from build123d import *

# Parameters (mm, degrees)
SKETCH_1_R          = 28.4
EXTRUDE_1_DEPTH     = 6
SKETCH_2_R          = 15
EXTRUDE_2_DEPTH     = 20.4
SKETCH_3_R          = 7
CUT_EXTRUDE_1_DEPTH = 54.68780863
SKETCH_4_W          = 5
SKETCH_4_H          = 2.1
CUT_EXTRUDE_2_DEPTH = 54.68780863
SKETCH_5_R          = 2.6
CUT_EXTRUDE_3_DEPTH = 52.005693755


with BuildPart() as part:
    # 草图1 → 凸台-拉伸1 (new body)
    with BuildSketch(Plane.XY):
        with Locations((0, 8.733014899)):
            Circle(SKETCH_1_R)
    extrude(amount=EXTRUDE_1_DEPTH)

    # 草图2 → 凸台-拉伸2 (add)
    with BuildSketch(Plane.XY.offset(6)):
        with Locations((0, 8.733014899)):
            Circle(SKETCH_2_R)
    extrude(amount=EXTRUDE_2_DEPTH)

    # 草图3 → 切除-拉伸1 (cut, through all)
    with BuildSketch(Plane.XY.offset(26.4)):
        with Locations((0, 8.733014899)):
            Circle(SKETCH_3_R)
    extrude(amount=-CUT_EXTRUDE_1_DEPTH, mode=Mode.SUBTRACT)

    # 草图4 → 切除-拉伸2 (cut, through all)
    with BuildSketch(Plane.XY.offset(26.4)):
        with Locations((0, 16.321363314)):
            Rectangle(SKETCH_4_W, SKETCH_4_H)
    extrude(amount=-CUT_EXTRUDE_2_DEPTH, mode=Mode.SUBTRACT)

    # 草图5 → 切除-拉伸3 (cut, through all)
    with BuildSketch(Plane.XY.offset(6)):
        with Locations((0, 32.483014899)):
            Circle(SKETCH_5_R)
        with Locations((20.56810334, 20.608014899)):
            Circle(SKETCH_5_R)
        with Locations((20.56810334, -3.141985101)):
            Circle(SKETCH_5_R)
        with Locations((0, -15.016985101)):
            Circle(SKETCH_5_R)
        with Locations((-20.56810334, -3.141985101)):
            Circle(SKETCH_5_R)
        with Locations((-20.56810334, 20.608014899)):
            Circle(SKETCH_5_R)
    extrude(amount=-CUT_EXTRUDE_3_DEPTH, mode=Mode.SUBTRACT)


solid = part.part
Design review of the part built by this model. Coordinates are the model's own, in mm. A direction names the side the tool comes from. Give positions to 0.01 mm unless a question says otherwise; leave off trailing zeros. Loops run counter-clockwise (first coordinate to the right, second up) from the corner with the lowest first, then second, coordinate; pieces in that order, holes last. Notation, with made-up numbers: M 17.25,-21 L 31.25,-21 A36 ccw 31.25,13 Z; hole C 64,66 d3. An arc over 180 degrees is marked long. Answer as a JSON object with one key per item and string values.
Item 1: Wall thickness on line 1 along Y through (x, z) = (0, 3.4); line 2 along Y through (x, z) = (0, 7.5); line 3 along X through (y, z) = (21, 2): over which ranges is each line inside the solid? List them lowest first.
Output values:
{"line 1": "y = -19.67 to -17.62, -12.42 to 1.73, 17.37 to 29.88, 35.08 to 37.13", "line 2": "y = -6.27 to 1.73, 17.37 to 23.73", "line 3": "x = -25.61 to -23.14, -18 to 18, 23.14 to 25.61"}
Item 2: We need section C-C (x = 6). State the section outline as (y, z) points, and give its area (3 significant figures).
Output values:
{"outline": "M -19.03,0 L 5.13,0 L 5.13,26.4 L -5.01,26.4 L -5.01,6 L -19.03,6 Z; M 12.34,0 L 36.49,0 L 36.49,6 L 22.48,6 L 22.48,26.4 L 12.34,26.4 Z", "area": "704 mm2"}
Item 3: Mouldability with a two-part tool opening along X and no side actions: class faces 4 (the face through (-3.3, -5.9, 16.1)), 5 (the face through (6, 3, 0)), 6 (the face through (0, 17.371, 13)) as pulls with the +X half, pulls with the -X half, needs draft (parallel to the pull), parting line crosses it, or undercut.
Output values:
{"face 4": "parting line crosses it", "face 5": "needs draft", "face 6": "undercut"}
Item 4: For P1, Ø8, axis at x = -8.5, z = 22.5, coming from the -Y side; P2, Ø3, axis at y = 1, z = 6, coming from the +X side; P3, Ø8, axis at y = 23.5, z = 12.5, coming from the +X side; P4, Ø1.5, axis at x = -9.5, y = -3.5, coming from the +Z side, all flat-tipped, find the tip position at first contact; note any pin that passes through.
Output values:
{"P1": "stops at y = -5.58", "P2": "stops at x = 27.71", "P3": "stops at x = 10.44", "P4": "stops at z = 26.4"}
Item 5: We need section A-A (x = 0). State the section outline as (y, z) points.
Output values:
{"outline": "M -19.67,0 L -17.62,0 L -17.62,6 L -19.67,6 Z; M -12.42,0 L 1.73,0 L 1.73,26.4 L -6.27,26.4 L -6.27,6 L -12.42,6 Z; M 17.37,0 L 29.88,0 L 29.88,6 L 23.73,6 L 23.73,26.4 L 17.37,26.4 Z; M 35.08,0 L 37.13,0 L 37.13,6 L 35.08,6 Z"}
Item 6: We need section D-D (z = 2.75). State the section outline as (x, y) points, and give its area (3 significant figures).
Output values:
{"outline": "C 0,8.73 d56.8; hole C -20.57,-3.14 d5.2; hole C -20.57,20.61 d5.2; hole C 0,-15.02 d5.2; hole C 0,32.48 d5.2; hole M -2.5,15.27 A7 ccw long 2.5,15.27 L 2.5,17.37 L -2.5,17.37 Z; hole C 20.57,-3.14 d5.2; hole C 20.57,20.61 d5.2", "area": "2,240 mm2"}
Item 7: Machinability: for faces 1 (the face through (3, 2, 26.4)), 2 (the face through (2.5, 16, 13)), 3 (the face through (12, -3, 6)), which of the approach directions +Z, -Z, +X, -X, +Y, -Y give a long, thin tool a straight path to every point of the face, cutting with its end or side? Answer none if there is none.
Output values:
{"face 1": "+Z, +X, -X, +Y, -Y", "face 2": "+Z, -Z", "face 3": "+Z"}
Item 8: We need section B-B (y = 11.5). State the section outline as (x, z) points, and give its area (3 significant figures).
Output values:
{"outline": "M -28.26,0 L -6.43,0 L -6.43,26.4 L -14.74,26.4 L -14.74,6 L -28.26,6 Z; M 6.43,0 L 28.26,0 L 28.26,6 L 14.74,6 L 14.74,26.4 L 6.43,26.4 Z", "area": "601 mm2"}
